Could you check a few things on this model? Use its own coordinates, in mm. Give positions to 0.01 mm unless a question says otherwise; leave off trailing zeros. Loops run counter-clockwise (first coordinate to the right, second up) from the corner with the lowest first, then second, coordinate; pieces in that order, holes last. Notation, with made-up numbers: (72.25, 30.5) - (84.25, 30.5) arc R21 ccw to (84.25, 44.5) - close; hole circle Ø6 at (64, 6.5). An arc over 180 degrees is marked (long way). One line per item, written item: value. Start each with the question number.
Q1. If I drill on line 1 (Y direction, x = 241.46, z = -0.2); line 2 (X direction, y = 0.25, z = -0.35); line 3 (X direction, y = 1.25, z = -0.6), over which ranges is the centre line in solid material (lowest first)? Write a range as from..to.
Q2. I want a section at A-A (y = 0). Please give me the cut outline in (x, z).
Q3. If we mould it in two halves opening along X, with no side actions, what happens to faces 1 (the face through (126, 0, 2.5)), 2 (the face through (244.56, 0.98, -0.04)), 3 (the face through (248.96, 0.16, 0.04))? For each: released by +X, released by -X, zero draft, split by the parting line, or undercut.
Q4. I want a section at B-B (z = 0.95). Please give me the cut outline in (x, y), then the cut area to 3 significant figures.
```python
from build123d import *

# Parameters (mm, degrees)
SKETCH1_R           = 3.25
BOSS_EXTRUDE1_DEPTH = 2.5


with BuildPart() as part:
    # Sketch1 → Boss-Extrude1 (new, symmetric)
    with BuildSketch(Plane.XY):
        with BuildLine():
            Line((0, 7.5), (241.46, 7.5))
            ThreePointArc((241.46, 7.5), (248.96, 0), (241.46, -7.5))
            Line((241.46, -7.5), (0, -7.5))
            Line((0, -7.5), (0, 7.5))
        make_face()
        with Locations((241.46, 0)):
            Circle(SKETCH1_R, mode=Mode.SUBTRACT)
    extrude(amount=BOSS_EXTRUDE1_DEPTH, both=True)


solid = part.part
```
Worked answers:
1. line 1: y = -7.5..-3.25, 3.25..7.5
1. line 2: x = 0..238.22, 244.7..248.96
1. line 3: x = 0..238.46, 244.46..248.86
2. outline: (0, -2.5) - (238.21, -2.5) - (238.21, 2.5) - (0, 2.5) - close; (244.71, -2.5) - (248.96, -2.5) - (248.96, 2.5) - (244.71, 2.5) - close
3. face 1: zero draft
3. face 2: undercut
3. face 3: released by +X
4. outline: (0, -7.5) - (241.46, -7.5) arc R7.5 ccw to (241.46, 7.5) - (0, 7.5) - close; hole circle Ø6.5 at (241.46, 0)
4. area: 3,680 mm²
